from build123d import *

# Parameters (mm, degrees)
F0_W     = 39.1890458631
F0_H     = 39.1890458631
F0_R     = 3.175
F1_DEPTH = 127
F2_DEPTH = 101.6
F3_DEPTH = 76.2
F4_DEPTH = 50.8
F5_DEPTH = 25.4


with BuildPart() as f1:
    # F0 (on Top) → F1 (new body)
    with BuildSketch(Plane.XY):
        Polygon((-22.6258061783, 22.6258061783), (8.2816198424, 30.9074260207), (-9.5627908906, 35.688821466), align=None)
        Polygon((-9.5627908906, 35.688821466), (8.2816198424, 30.9074260207), (26.1260305754, 26.1260305754), (30.9074260207, 8.2816198424), (35.688821466, -9.5627908906), (22.6258061783, -22.6258061783), (9.5627908906, -35.688821466), (24.345584767, -31.727783785), (39.6498591471, -5.2200029857), (31.727783785, 24.345584767), (5.2200029857, 39.6498591471), align=None)
        Polygon((-35.688821466, 9.5627908906), (-22.6258061783, 22.6258061783), (-9.5627908906, 35.688821466), (-24.345584767, 31.727783785), (-39.6498591471, 5.2200029857), (-31.727783785, -24.345584767), (-5.2200029857, -39.6498591471), (9.5627908906, -35.688821466), (-8.2816198424, -30.9074260207), (-26.1260305754, -26.1260305754), (-30.9074260207, -8.2816198424), align=None)
        Polygon((9.5627908906, -35.688821466), (22.6258061783, -22.6258061783), (-8.2816198424, -30.9074260207), align=None)
        Polygon((-30.9074260207, -8.2816198424), (-22.6258061783, 22.6258061783), (-35.688821466, 9.5627908906), align=None)
        Polygon((-8.2816198424, -30.9074260207), (-19.5945229316, -19.5945229316), (-30.9074260207, -8.2816198424), (-26.1260305754, -26.1260305754), align=None)
        Polygon((30.9074260207, 8.2816198424), (19.5945229316, 19.5945229316), (19.5945229316, -19.5945229316), (-19.5945229316, -19.5945229316), (-8.2816198424, -30.9074260207), (22.6258061783, -22.6258061783), align=None)
        Polygon((35.688821466, -9.5627908906), (30.9074260207, 8.2816198424), (22.6258061783, -22.6258061783), align=None)
        Polygon((8.2816198424, 30.9074260207), (19.5945229316, 19.5945229316), (30.9074260207, 8.2816198424), (26.1260305754, 26.1260305754), align=None)
        Polygon((-19.5945229316, 19.5945229316), (19.5945229316, 19.5945229316), (8.2816198424, 30.9074260207), (-22.6258061783, 22.6258061783), (-30.9074260207, -8.2816198424), (-19.5945229316, -19.5945229316), align=None)
        Rectangle(F0_W, F0_H)
        Circle(F0_R, mode=Mode.SUBTRACT)
        Circle(F0_R)
    extrude(amount=-F1_DEPTH)

    # F0 (on Top) → F2 (cut)
    with BuildSketch(Plane.XY):
        Polygon((-35.688821466, 9.5627908906), (-22.6258061783, 22.6258061783), (-9.5627908906, 35.688821466), (-24.345584767, 31.727783785), (-39.6498591471, 5.2200029857), (-31.727783785, -24.345584767), (-5.2200029857, -39.6498591471), (9.5627908906, -35.688821466), (-8.2816198424, -30.9074260207), (-26.1260305754, -26.1260305754), (-30.9074260207, -8.2816198424), align=None)
        Polygon((-9.5627908906, 35.688821466), (8.2816198424, 30.9074260207), (26.1260305754, 26.1260305754), (30.9074260207, 8.2816198424), (35.688821466, -9.5627908906), (22.6258061783, -22.6258061783), (9.5627908906, -35.688821466), (24.345584767, -31.727783785), (39.6498591471, -5.2200029857), (31.727783785, 24.345584767), (5.2200029857, 39.6498591471), align=None)
    extrude(amount=-F2_DEPTH, mode=Mode.SUBTRACT)

    # F0 (on Top) → F3 (cut)
    with BuildSketch(Plane.XY):
        Polygon((-8.2816198424, -30.9074260207), (-19.5945229316, -19.5945229316), (-30.9074260207, -8.2816198424), (-26.1260305754, -26.1260305754), align=None)
        Polygon((9.5627908906, -35.688821466), (22.6258061783, -22.6258061783), (-8.2816198424, -30.9074260207), align=None)
        Polygon((35.688821466, -9.5627908906), (30.9074260207, 8.2816198424), (22.6258061783, -22.6258061783), align=None)
        Polygon((8.2816198424, 30.9074260207), (19.5945229316, 19.5945229316), (30.9074260207, 8.2816198424), (26.1260305754, 26.1260305754), align=None)
        Polygon((-22.6258061783, 22.6258061783), (8.2816198424, 30.9074260207), (-9.5627908906, 35.688821466), align=None)
        Polygon((-30.9074260207, -8.2816198424), (-22.6258061783, 22.6258061783), (-35.688821466, 9.5627908906), align=None)
    extrude(amount=-F3_DEPTH, mode=Mode.SUBTRACT)

    # F0 (on Top) → F4 (cut)
    with BuildSketch(Plane.XY):
        Polygon((-19.5945229316, 19.5945229316), (19.5945229316, 19.5945229316), (8.2816198424, 30.9074260207), (-22.6258061783, 22.6258061783), (-30.9074260207, -8.2816198424), (-19.5945229316, -19.5945229316), align=None)
        Polygon((30.9074260207, 8.2816198424), (19.5945229316, 19.5945229316), (19.5945229316, -19.5945229316), (-19.5945229316, -19.5945229316), (-8.2816198424, -30.9074260207), (22.6258061783, -22.6258061783), align=None)
    extrude(amount=-F4_DEPTH, mode=Mode.SUBTRACT)

    # F0 (on Top) → F5 (cut)
    with BuildSketch(Plane.XY):
        Rectangle(F0_W, F0_H)
        Circle(F0_R, mode=Mode.SUBTRACT)
    extrude(amount=-F5_DEPTH, mode=Mode.SUBTRACT)


solid = f1.part
The model under review builds one solid part; all positions refer to its coordinate system, in mm. A direction names the side the tool comes from. Round coordinates to 2 decimals unless told otherwise and drop trailing zeros. Loops run counter-clockwise (first coordinate to the right, second up) from the corner with the lowest first, then second, coordinate; pieces in that order, holes last. Notation, with made-up numbers: (-23.75, -30) -> (27.25, -30) arc R16 ccw to (27.25, -5) -> close; hole circle Ø2 at (22.5, 26). An arc over 180 degrees is marked (long way). Write item = value, one per line. Start each with the question number.
Item 1: To check wall thickness, follow L1, parallel to X at y = -13.5, z = -31; L2, parallel to Z at x = -8.5, y = -24; L3, parallel to Z at x = -32.5, y = -17. State the ranges of each line that lie inside material, in increasing order.
Item 2: Take a section at C-C on x = 0. Give the boundary of the cut face in (y, z) (3 decimals), plus the area to 3 significant figures.
Item 3: Take a section at A-A on z = -54. Give the boundary of the cut face in (x, y), plus the area to 3 significant figures.
Item 4: For faces 4 (the flat face through (29, -7, -76.2)), 5 (the flat face through (8.032, 30.974, -88.722)), 6 (the flat face through (-7, 29, -76.2)), list the 3-axis set-ups (+Z, -Z, +X, -X, +Y, -Y) from which the entire face can be reached by the end or side of a thin tool; tool diameter is ignored.
Item 5: Take a section at D-D on z = -81. Give the boundary of the cut face in (x, y), plus the area to 3 significant figures.
Item 6: Insertion check: pin 1 (7 mm diameter, centred on x = -19.5, y = -24.5, fed in from +Z); pin 2 (15 mm diameter, centred on x = -6.5, y = 0, fed in from +Z); pin 3 (6 mm diameter, centred on x = -17, z = -79.5, fed in from -Y); pin 4 (7 mm diameter, centred on x = 20.5, y = 22, fed in from +Z). Each pin has a flat end and moves straight along its axis. Give the tip position at first contact, or say it passes through.
Item 7: Take a section at B-B on y = 34. Give the boundary of the cut face in (x, z).
Item 8: Mouldability with a two-part tool opening along X and no side actions: class faces 1 (the flat face through (22, 22, -76.2)), 2 (the flat face through (35.744, 9.356, -114.122)), 3 (the flat face through (-22.81, 22.44, -88.72)) as released by +X, released by -X, zero draft, split by the parting line, or undercut.
Result:
q1.L1 = -19.59 to 19.59
q1.L2 = -127 to -50.8
q1.L3 = -127 to -101.6
q2.outline = (-38.251, -127) -> (38.251, -127) -> (38.251, -101.6) -> (33.126, -101.6) -> (33.126, -76.2) -> (28.688, -76.2) -> (28.688, -50.8) -> (19.595, -50.8) -> (19.595, -25.4) -> (3.175, -25.4) -> (3.175, 0) -> (-3.175, 0) -> (-3.175, -25.4) -> (-19.595, -25.4) -> (-19.595, -50.8) -> (-28.688, -50.8) -> (-28.688, -76.2) -> (-33.126, -76.2) -> (-33.126, -101.6) -> (-38.251, -101.6) -> close
q2.area = 6,240 mm²
q3.outline = (-30.91, -8.28) -> (-8.28, -30.91) -> (22.63, -22.63) -> (30.91, 8.28) -> (8.28, 30.91) -> (-22.63, 22.63) -> close
q3.area = 2,660 mm²
q4.face_4 = +Z, +X, -Y
q4.face_5 = +Z, +X, +Y
q4.face_6 = +Z, -X, +Y
q5.outline = (-35.69, 9.56) -> (-26.13, -26.13) -> (9.56, -35.69) -> (35.69, -9.56) -> (26.13, 26.13) -> (-9.56, 35.69) -> close
q5.area = 3,550 mm²
q6.pin_1 = -50.8
q6.pin_2 = 0
q6.pin_3 = -29.38
q6.pin_4 = -25.4
q7.outline = (-15.87, -127) -> (15.01, -127) -> (15.01, -101.6) -> (-3.26, -101.6) -> (-3.26, -76.2) -> (-11.25, -76.2) -> (-11.25, -101.6) -> (-15.87, -101.6) -> close
q8.face_1 = zero draft
q8.face_2 = released by +X
q8.face_3 = released by -X
